Could you check a few things on this model? Use its own coordinates, in mm. Face numbers are marked on the shaded views. A direction names the side the tool comes from. Give positions to 0.01 mm unless a question says otherwise; leave off trailing zeros. Loops run counter-clockwise (first coordinate to the right, second up) from the corner with the lowest first, then second, coordinate; pieces in that order, holes last. Notation, with made-up numbers: M -3,50 L 42,50 A13 ccw 42,58 Z; hole C 58.5,11.25 d3. An arc over 180 degrees is marked long. Return JSON: item names as keys, results as strings. Group by question number.
1. If we section it at B-B (y = 0): Write out the boundary of the cut face in (x, z) (3 decimals).
2. If we section it at D-D (x = 12.7): Write out the boundary of the cut face in (y, z) (3 decimals), plus the area to 3 significant figures.
3. For pin 1 (2 mm diameter, centred on x = -10, y = 5.5, fed in from -Z); pin 2 (5.5 mm diameter, centred on x = -5.5, z = -13.5, fed in from +Y), each with a flat end and sliding along its axis, tell me the tip position at first contact or that it passes through.
4. For the marked faces 1 and 2, which set-ups out of +Z, -Z, +X, -X, +Y, -Y let a thin tool reach every point of the face, with its end or its side?
5. If we section it at C-C (z = -8.75): Write out the boundary of the cut face in (x, y), plus the area to 3 significant figures.
6. If we section it at A-A (x = 0): Write out the boundary of the cut face in (y, z) (3 decimals).
7. Please list where these lines run through material, in increasing order: line 1 (Y direction, x = 5.75, z = 1.9) (3 decimals); line 2 (Z direction, x = 3.5, y = -19) (3 decimals); line 3 (Y direction, x = 9.5, z = -7.25).
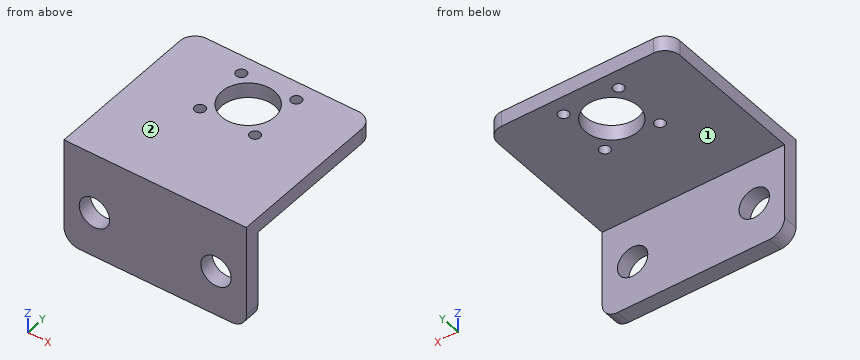
```python
from build123d import *

# Parameters (mm, degrees)
SKETCH1_W                   = 38.1
SKETCH1_H                   = 35.433
SKETCH1_R                   = 5.55
BOSS_EXTRUDE1_DEPTH         = 3.175
SKETCH3_W                   = 38.1
SKETCH3_H                   = 3.175
BOSS_EXTRUDE2_DEPTH         = 19.05
FILLET1_R                   = 3.175
M2_CLEARANCE_HOLE1_D        = 2.2
F_1_4_0_25_DIAMETER_HOLE1_D = 6.35


with BuildPart() as part:
    # Sketch1 → Boss-Extrude1 (new body)
    with BuildSketch(Plane.XY):
        with Locations((0, -8.1915)):
            Rectangle(SKETCH1_W, SKETCH1_H)
        Circle(SKETCH1_R, mode=Mode.SUBTRACT)
    extrude(amount=BOSS_EXTRUDE1_DEPTH)

    # Sketch3 → Boss-Extrude2 (add)
    with BuildSketch(Plane(origin=(0, 0, 0), x_dir=(-1, 0, 0), z_dir=(0, 0, -1))):
        with Locations((0, -24.3205)):
            Rectangle(SKETCH3_W, SKETCH3_H)
    extrude(amount=BOSS_EXTRUDE2_DEPTH)

    # Fillet1
    fillet1_edges = [part.edges().sort_by_distance(p)[0] for p in [
        (-19.05, -24.3205, -19.05),
        (19.05, -24.3205, -19.05),
        (-19.05, 9.525, 1.5875),
        (19.05, 9.525, 1.5875),
    ]]
    fillet(fillet1_edges, radius=FILLET1_R)

    # M2 Clearance Hole1 (through all)
    with Locations(Plane(origin=(0, -25.908, 3.175), x_dir=(1, 0, 0), z_dir=(0, 0, 1))):
        with Locations((5.75, 31.658), (-5.75, 31.658), (5.75, 20.158), (-5.75, 20.158)):
            Hole(M2_CLEARANCE_HOLE1_D / 2)

    # 1/4 (0.25) Diameter Hole1 (through all)
    with Locations(Plane(origin=(0, -22.733, 0), x_dir=(1, 0, 0), z_dir=(0, 1, 0))):
        with Locations((-12.7, 9.525), (12.7, 9.525)):
            Hole(F_1_4_0_25_DIAMETER_HOLE1_D / 2)


solid = part.part
```
Answer:
{
 "1": {"outline": "M -19.05,0 L -5.55,0 L -5.55,3.175 L -19.05,3.175 Z; M 5.55,0 L 19.05,0 L 19.05,3.175 L 5.55,3.175 Z"},
 "2": {"outline": "M -25.908,-19.05 L -22.733,-19.05 L -22.733,-12.7 L -25.908,-12.7 Z; M -25.908,-6.35 L -22.733,-6.35 L -22.733,0 L 9.525,0 L 9.525,3.175 L -25.908,3.175 Z", "area": "153 mm²"},
 "3": {"pin 1": "stops at z = 0", "pin 2": "stops at y = -22.73"},
 "4": {"face 1": "-Z, +X, -X, +Y", "face 2": "+Z, +X, -X, +Y, -Y"},
 "5": {"outline": "M -19.05,-25.91 L -15.78,-25.91 L -15.78,-22.73 L -19.05,-22.73 Z; M -9.62,-25.91 L 9.62,-25.91 L 9.62,-22.73 L -9.62,-22.73 Z; M 15.78,-25.91 L 19.05,-25.91 L 19.05,-22.73 L 15.78,-22.73 Z", "area": "81.9 mm²"},
 "6": {"outline": "M -25.908,-19.05 L -22.733,-19.05 L -22.733,0 L -5.55,0 L -5.55,3.175 L -25.908,3.175 Z; M 5.55,0 L 9.525,0 L 9.525,3.175 L 5.55,3.175 Z"},
 "7": {"line 1": "y = -25.908 to -6.85, -4.65 to 4.65, 6.85 to 9.525", "line 2": "z = 0 to 3.175", "line 3": "y = -25.91 to -22.73"}
}
